Autodesk Inventor part; units mm, degrees
ref_plane "YZ Plane" through (0, 0, 0) normal (1, 0, 0) x (0, 1, 0)
ref_plane "XZ Plane" through (0, 0, 0) normal (0, 1, 0) x (-1, 0, 0)
ref_plane "XY Plane" through (0, 0, 0) normal (0, 0, 1) x (1, 0, 0)
sketch "Sketch1" plane through (0, 0, 0) normal (0, 0, 1) x (1, 0, 0)
  line L0 (10, -10) -> (-10, -10)
  line L1 (-10, -10) -> (-10, 10)
  line L2 (-10, 10) -> (10, 10)
  line L3 (10, 10) -> (10, -10)
  circle A0 centre (0, 5) radius 1.2
  circle A1 centre (0, -5) radius 1.2
  circle A2 centre (0, 0) radius 3
  dimension "d0" = 10
  dimension "d1" = 10
  dimension "d2" = 10
  dimension "d3" = 10
  dimension "d4" = 5
  dimension "d5" = 5
  dimension "d6" = 2.4
  dimension "d7" = 2.4
  dimension "d8" = 6
extrude "Extrusion1" add sketch "Sketch1" along normal blind 5
sketch "Sketch2" plane through (0, 0, 5) normal (0, 0, 1) x (1, 0, 0)
  line L0 (0, 0) -> (-1.3346, -1.3533)
  circle A0 centre (6, -6) radius 2.5
  circle A1 centre (6, 6) radius 2.5
  line L1 (10, -10) -> (10, 10)
  line L2 (-10, -10) -> (10, -10)
  line L3 (10, 10) -> (-10, 10)
  dimension "d34" = 4
  dimension "d35" = 4
  dimension "d36" = 4
  dimension "d37" = 4
  dimension "d38" = 5
  dimension "d39" = 5
extrude "Extrusion2" cut sketch "Sketch2" against normal blind 1
sketch "Sketch7" plane through (0, 0, 0) normal (0, 0, -1) x (-1, 0, 0)
  circle A0 centre (-6, 6) radius 2.5
  circle A1 centre (-6, 6) radius 1.375
  circle A2 centre (-6, -6) radius 2.5
  circle A3 centre (-6, -6) radius 1.375
  point P0 (0, 0)
  dimension "d40" = 2.75
  dimension "d41" = 2.75
extrude "Extrusion6" cut sketch "Sketch7" against normal blind 5 contours A1 | A3
sketch "Sketch8" plane through (0, 0, 5) normal (0, 0, 1) x (1, 0, 0)
  line L0 (10, 10) -> (-10, 10)
  line L1 (10, 10) -> (2.5, 10)
  line L2 (2.5, 10) -> (2.5, 2.5)
  line L3 (2.5, 2.5) -> (10, 2.5)
  line L4 (10, 2.5) -> (10, 10)
  line L5 (10, -10) -> (10, 10)
  line L6 (10, -10) -> (2.5, -10)
  line L7 (2.5, -10) -> (2.5, -2.5)
  line L8 (2.5, -2.5) -> (10, -2.5)
  line L9 (10, -2.5) -> (10, -10)
  line L10 (10, -2.5) -> (5, -2.5)
  line L11 (5, -2.5) -> (5, 2.5)
  line L12 (5, 2.5) -> (10, 2.5)
  line L13 (10, 2.5) -> (10, -2.5)
  circle A0 centre (6, 6) radius 2.5
  circle A1 centre (6, 6) radius 2.5
  circle A2 centre (6, -6) radius 2.5
  circle A3 centre (6, -6) radius 2.5
  point P0 (0, 0)
  point P1 (2.5, 10)
  dimension "d44" = 7.5
  dimension "d45" = 7.5
  dimension "d46" = 7.5
  dimension "d47" = 7.5
  dimension "d48" = 5
extrude "Extrusion7" add sketch "Sketch8" along normal blind 2
sketch "Sketch9" plane through (0, 0, 0) normal (0, 0, -1) x (-1, 0, 0)
  circle A0 centre (-6, 6) radius 1.375
  circle A1 centre (-6, 6) radius 2.5
  circle A2 centre (-6, -6) radius 1.375
  circle A3 centre (-6, -6) radius 2.5
  point P0 (0, 0)
  dimension "d51" = 5
  dimension "d52" = 5
extrude "Extrusion8" cut sketch "Sketch9" against normal blind 2.5 contours A0 | A1 | A2 | A3
sketch "Sketch10" plane through (0, 0, 0) normal (0, 0, -1) x (-1, 0, 0)
  line L0 (-2.5, 10) -> (10, 10)
  line L1 (10, -10) -> (-2.5, -10)
  line L2 (10, 10) -> (5, 10)
  line L3 (5, 10) -> (5, -10)
  line L4 (5, -10) -> (10, -10)
  line L5 (10, -10) -> (10, 10)
  line L6 (5, 10) -> (2.5, 10)
  line L7 (2.5, 10) -> (2.5, 5)
  line L8 (2.5, 5) -> (5, 5)
  line L9 (5, 5) -> (5, 10)
  line L10 (5, -10) -> (2.5, -10)
  line L11 (2.5, -10) -> (2.5, -5)
  line L12 (2.5, -5) -> (5, -5)
  line L13 (5, -5) -> (5, -10)
  point P0 (0, 0)
  point P1 (2.5, 10)
  dimension "d55" = 5
  dimension "d56" = 2.5
  dimension "d57" = 5
  dimension "d58" = 5
  dimension "d59" = 2.5
extrude "Extrusion9" cut sketch "Sketch10" against normal blind 10
sketch "Sketch12" plane through (6, -6, 4) normal (0, 0, 1) x (1, 0, 0)
  circle A0 centre (0, 0) radius 1.375
  circle A1 centre (0, 0) radius 2.5
  circle A2 centre (0, 12) radius 2.5
  circle A3 centre (0, 12) radius 1.375
  circle A4 centre (0, 12) radius 2.5
  point P0 (-6, 6)
extrude "Extrusion11" add sketch "Sketch12" along normal blind 1.5
sketch "Sketch13" plane through (0, 0, 5) normal (0, 0, 1) x (1, 0, 0)
  point P0 (0, 0)
sketch "Sketch14" plane through (0, 0, 5) normal (0, 0, 1) x (1, 0, 0)
  line L0 (-2.5, -5) -> (-2.5, -10)
  line L1 (-2.5, -10) -> (2.5, -10)
  line L2 (2.5, -10) -> (2.5, -2.5)
  line L3 (2.5, -2.5) -> (5, -2.5)
  line L4 (5, -2.5) -> (5, 2.5)
  line L5 (5, 2.5) -> (2.5, 2.5)
  line L6 (2.5, 2.5) -> (2.5, 10)
  line L7 (2.5, 10) -> (-2.5, 10)
  line L8 (-2.5, 10) -> (-2.5, 5)
  line L9 (-2.5, 5) -> (-5, 5)
  line L10 (-5, 5) -> (-5, -5)
  line L11 (-5, -5) -> (-2.5, -5)
  circle A0 centre (0, 0) radius 3
  circle A1 centre (0, -5) radius 1.2
  circle A2 centre (0, 5) radius 1.2
  circle A3 centre (0, -5) radius 1.95
  circle A4 centre (0, 5) radius 1.95
  dimension "d80" = 3.9
  dimension "d81" = 3.9
extrude "Extrusion12" add sketch "Sketch14" along normal blind 2 contours L11 L10 L9 L8 L7 L6 L5 L4 L3 L2 L1 L0
sketch "Sketch15" plane through (-5, -5, 0) normal (-1, 0, 0) x (0, 0, 1)
  line L0 (0, 10) -> (7, 10)
  line L1 (0, 0) -> (0, 10)
  line L2 (0, 0) -> (7, 0)
  line L3 (7, 10) -> (7, 0)
  point P0 (0, 5)
extrude "Extrusion13" cut sketch "Sketch15" against normal blind 0.5
equation "\"d7\" = d6"
equation "\"d39\" = d38"
equation "\"d45\" = d44"
equation "\"d46\" = d45"
equation "\"d52\" = d51"
equation "\"d81\" = d80"
properties part number "MotorMount" material "Stainless Steel"
Build history of the part. All positions in model axes, mm. A direction names the side the tool comes from. Give positions to 0.01 mm unless a question says otherwise; leave off trailing zeros. Order: outer loops, then holes, each group sorted by start corner. A loop starts at its lowest first (then second) coordinate and runs counter-clockwise, first axis right, second up. Notation, with made-up numbers: M -36.5,55.25 L -29.5,55.25 A29 ccw -29.5,87.25 Z; hole C 84.25,-20 d5. An arc over 180 degrees is marked long. Put each result on its own line as item: value.
Item 1: Which spindle directions (+Z, -Z, +X, -X, +Y, -Y) get a long thin tool onto all of the face, cutting with end or side? Do faces 1 (the face through (4.9, 4.9, 2.5)), 2 (the face through (-2.5, 8, 3)), 3 (the face through (4, 0, 0)), 4 (the face through (-2.5, -7, 3)), 5 (the face through (7.1, -7.1, 5.5)). Say none if no direction does.
Results are:
face 1: -Z
face 2: +Z, -Z, -X, +Y
face 3: -Z, +X, -X, +Y, -Y
face 4: +Z, -Z, -X, -Y
face 5: +Z
Item 2: Cut at D-D on z = 4.5. Write the cut outline in (x, y) (3 decimals), then the cut area to 3 significant figures.
Results are:
outline: M -4.5,-5 L -2.5,-5 L -2.5,-10 L 10,-10 L 10,10 L -2.5,10 L -2.5,5 L -4.5,5 Z; hole C 0,0 d6; hole C 0,-5 d2.4; hole C 0,5 d2.4; hole C 6,-6 d2.75; hole C 6,6 d2.75
area: 221 mm2
Item 3: Drop flat-ended pins along their axis: pin 1 Ø2.5 at (x, y) = (7, 6.5) entering from +Z; pin 2 Ø4.5 at (x, y) = (6, 6) entering from -Z; pin 3 Ø1.5 at (y, z) = (6.5, 4.5) entering from -X. Give the stop position or say it passes through.
Results are:
pin 1: z = 5.5
pin 2: z = 2.5
pin 3: x = -2.5
Item 4: Pull direction Y, two halves, no side cores. Call faces 6 (the face through (-4.5, 0, 3)), 7 (the face through (7.1, 4.9, 5.5)), 8 (the face through (-4, -5, 3)): +Y half, -Y half, draft (parallel to the pull), parting line (faces both ways), or undercut.
Results are:
face 6: draft
face 7: undercut
face 8: -Y half
Item 5: Cut at A-A on x = 6. Write the cut outline in (y, z) (3 decimals).
Results are:
outline: M -10,0 L -8.5,0 L -8.5,2.5 L -7.375,2.5 L -7.375,5.5 L -8.5,5.5 L -8.5,7 L -10,7 Z; M -4.625,2.5 L -3.5,2.5 L -3.5,0 L 3.5,0 L 3.5,2.5 L 4.625,2.5 L 4.625,5.5 L 3.5,5.5 L 3.5,7 L -3.5,7 L -3.5,5.5 L -4.625,5.5 Z; M 7.375,2.5 L 8.5,2.5 L 8.5,0 L 10,0 L 10,7 L 8.5,7 L 8.5,5.5 L 7.375,5.5 Z
Item 6: Cut at B-B on y = 0. Write the cut outline in (x, z).
Results are:
outline: M -4.5,0 L -3,0 L -3,7 L -4.5,7 Z; M 3,0 L 10,0 L 10,7 L 3,7 Z
Item 7: Wall check: probe 1 along Y at (x, z) = (6, 3.5) (3 decimals); probe 2 along Y at (x, z) = (6, 6.25); probe 3 along Y at (x, z) = (2.75, 5.5). Give the ranges that are in metal, low to high.
Results are:
probe 1: -10 to -7.375, -4.625 to 4.625, 7.375 to 10
probe 2: -10 to -8.5, -3.5 to 3.5, 8.5 to 10
probe 3: -10 to -1.2, 1.2 to 10
Item 8: Cut at C-C on x = 0. Write the cut outline in (y, z), then the cut area to 3 significant figures.
Results are:
outline: M -10,0 L -6.2,0 L -6.2,5 L -6.95,5 L -6.95,7 L -10,7 Z; M -3.8,0 L -3,0 L -3,7 L -3.05,7 L -3.05,5 L -3.8,5 Z; M 3,0 L 3.8,0 L 3.8,5 L 3.05,5 L 3.05,7 L 3,7 Z; M 6.2,0 L 10,0 L 10,7 L 6.95,7 L 6.95,5 L 6.2,5 Z
area: 58.4 mm2
